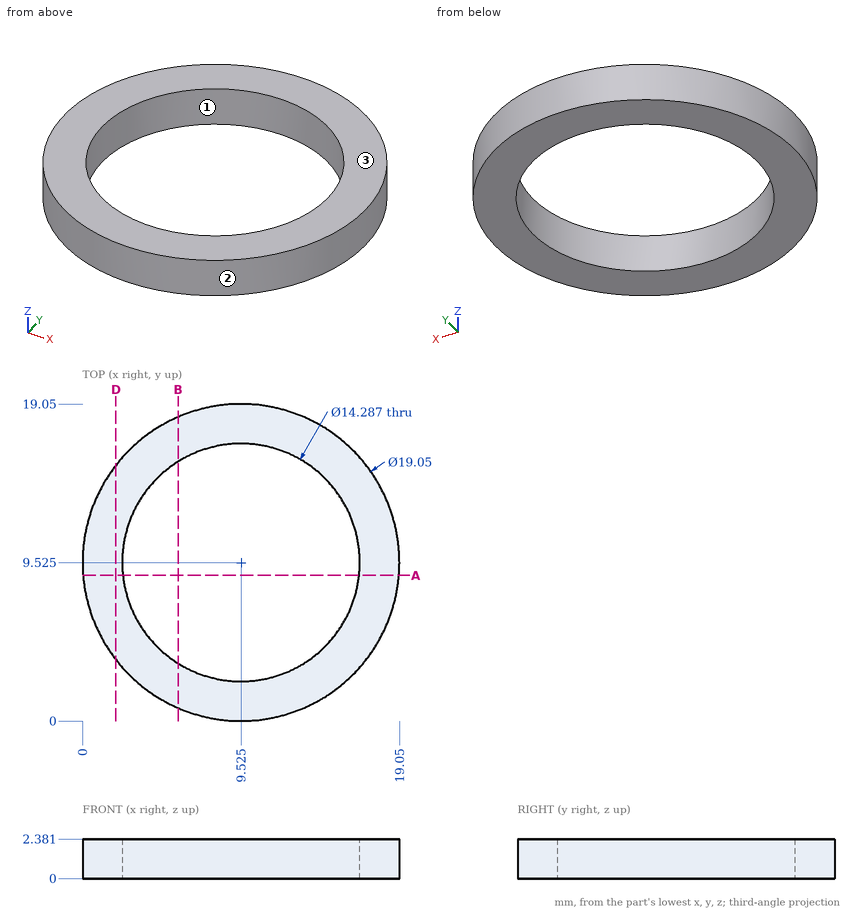
Print and shaded views of the part. All mm, measured from the part's lowest x, y and z. Coordinates: 2 decimals unless noted, no trailing zeros. Order: outer loops, then holes, each group sorted by start corner. A loop starts at its lowest first (then second) coordinate and runs counter-clockwise, first axis right, second up.
(1) Slice it at D-D, the plane x = 2. Write the cut outline in (y, z) (1 decimal).
Check sheet entries:
outline: (3.7, 0) - (15.4, 0) - (15.4, 2.4) - (3.7, 2.4) - close
(2) Pin check, flat tip, straight feed: pin 1 Ø3 at (x, y) = (6, 12.5) entering from -Z. Stop position of the tip, or through.
Check sheet entries:
pin 1: passes through
(3) Pull direction X, two halves, no side cores. Call the marked faces 1, 2 and 3: pulls with the +X half, pulls with the -X half, needs draft (parallel to the pull), parting line crosses it, or undercut.
Check sheet entries:
face 1: undercut
face 2: parting line crosses it
face 3: needs draft
(4) Slice it at A-A, the plane y = 8.75. Write the cut outline in (x, z).
Check sheet entries:
outline: (0.03, 0) - (2.42, 0) - (2.42, 2.38) - (0.03, 2.38) - close; (16.63, 0) - (19.02, 0) - (19.02, 2.38) - (16.63, 2.38) - close
(5) Probe L1, parallel to X at y = 9.5, z = 0.65; L2, parallel to Y at x = 3.75, z = 1.1; L3, parallel to X at y = 6.25, z = 1.05 (1 decimal). List the from-to ranges inside material, lowest first.
Check sheet entries:
L1: x = 0 to 2.38, 16.67 to 19.05
L2: y = 1.95 to 5.32, 13.73 to 17.1
L3: x = 0.6 to 3.2, 15.9 to 18.5
(6) Slice it at B-B, the plane x = 5.75. Write the cut outline in (y, z).
Check sheet entries:
outline: (0.78, 0) - (3.46, 0) - (3.46, 2.38) - (0.78, 2.38) - close; (15.59, 0) - (18.27, 0) - (18.27, 2.38) - (15.59, 2.38) - close
